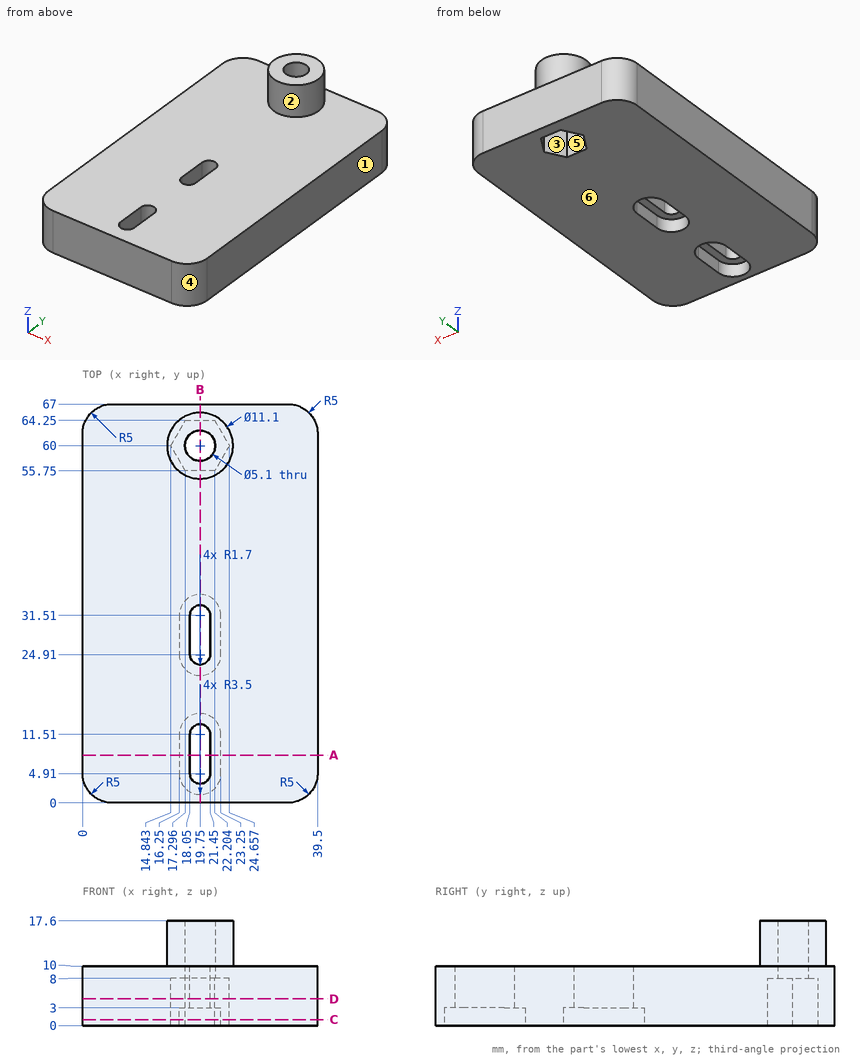
Could you check a few things on this drawing? It's one solid part, dimensions in mm from its lowest x, y, z. A direction names the side the tool comes from. Coordinates: 2 decimals unless noted, no trailing zeros. Write each loop counter-clockwise with the first axis right and the second up, starting at its lowest first coordinate (ties: lowest second). Pieces come first, ordered by that corner, then holes. Notation, with made-up numbers: M 66,31 L 79,31 A28 ccw 79,56 Z; hole C 3.25,71 d9. An arc over 180 degrees is marked long. Answer as CSV lines item,"result". Start each with the question number.
Q1. Suppose I cut it at C-C, the plane z = 1. List the corners of the cut face in (x, y) for me.
Q2. I need wall thicknesses on probe 1 along Y at (x, z) = (17, 2.5) (1 decimal); probe 2 along X at (y, z) = (60, 13); probe 3 along X at (y, z) = (27, 8). Which ranges of each line are inside material? Lowest first, please. Write a range as [from, to].
Q3. If we mould it in two halves opening along Y, with no side actions, what happens to the marked faces 3, 4, 5 and 6? For each: pulls with the +Y half, pulls with the -Y half, needs draft (parallel to the pull), parting line crosses it, or undercut.
Q4. Suppose I cut it at D-D, the plane z = 4.5. List the corners of the cut face in (x, y) for me.
Q5. Suppose I cut it at A-A, the plane y = 8. List the corners of the cut face in (x, z) for me, then the cut area to 3 significant figures.
Q6. For the marked faces 1 and 2, which set-ups out of +Z, -Z, +X, -X, +Y, -Y let a thin tool reach every point of the face, with its end or its side?
Q7. Will these pins go through, and if not, where does the flat tip stop? pin 1 Ø20 at (x, y) = (17, 21) entering from +Z; pin 2 Ø3.5 at (x, y) = (20, 31.5) entering from -Z.
Q8. Suppose I cut it at B-B, the plane x = 19.75. State how many separate pieces and enclosed holes the cut face has, then the cut area to 3 significant figures.
Entries:
1,outline,"M 0,5 A5 ccw 5,0 L 34.5,0 A5 ccw 39.5,5 L 39.5,62 A5 ccw 34.5,67 L 5,67 A5 ccw 0,62 Z; hole M 14.84,60 L 17.3,55.75 L 22.2,55.75 L 24.66,60 L 22.2,64.25 L 17.3,64.25 Z; hole M 16.25,4.91 A3.5 ccw 23.25,4.91 L 23.25,11.51 A3.5 ccw 16.25,11.51 Z; hole M 16.25,24.91 A3.5 ccw 23.25,24.91 L 23.25,31.51 A3.5 ccw 16.25,31.51 Z"
2,probe 1,"y = [0, 2.7], [13.7, 22.7], [33.7, 56.3], [63.7, 67]"
2,probe 2,"x = [14.2, 17.2], [22.3, 25.3]"
2,probe 3,"x = [0, 18.05], [21.45, 39.5]"
3,face 3,"undercut"
3,face 4,"pulls with the -Y half"
3,face 5,"undercut"
3,face 6,"needs draft"
4,outline,"M 0,5 A5 ccw 5,0 L 34.5,0 A5 ccw 39.5,5 L 39.5,62 A5 ccw 34.5,67 L 5,67 A5 ccw 0,62 Z; hole M 14.84,60 L 17.3,55.75 L 22.2,55.75 L 24.66,60 L 22.2,64.25 L 17.3,64.25 Z; hole M 18.05,4.91 A1.7 ccw 21.45,4.91 L 21.45,11.51 A1.7 ccw 18.05,11.51 Z; hole M 18.05,24.91 A1.7 ccw 21.45,24.91 L 21.45,31.51 A1.7 ccw 18.05,31.51 Z"
5,outline,"M 0,0 L 16.25,0 L 16.25,3 L 18.05,3 L 18.05,10 L 0,10 Z; M 21.45,3 L 23.25,3 L 23.25,0 L 39.5,0 L 39.5,10 L 21.45,10 Z"
5,area,"350 mm²"
6,face 1,"+Z, -Z, +X, +Y, -Y"
6,face 2,"+Z"
7,pin 1,"stops at z = 10"
7,pin 2,"stops at z = 3"
8,separate pieces,"4"
8,enclosed holes,"0"
8,area,"416 mm²"
